Geometry check sheet. Reference: the model listing, model coordinates, mm. A direction names the side the tool comes from. Coordinates: 2 decimals unless noted, no trailing zeros. Write each loop counter-clockwise with the first axis right and the second up, starting at its lowest first coordinate (ties: lowest second). Pieces come first, ordered by that corner, then holes. Notation, with made-up numbers: (-27, 15.25) -> (-23, 15.25) arc R16 ccw to (-23, 34.25) -> close; hole circle Ø9 at (84.25, 15.5). An arc over 180 degrees is marked (long way). One line per question, with ' | ' between items.
Autodesk Inventor part; units mm, degrees
ref_plane "YZ Plane" through (0, 0, 0) normal (1, 0, 0) x (0, 1, 0)
ref_plane "XZ Plane" through (0, 0, 0) normal (0, 1, 0) x (-1, 0, 0)
ref_plane "XY Plane" through (0, 0, 0) normal (0, 0, 1) x (1, 0, 0)
sketch "Sketch1" plane through (0, 0, 0) normal (0, 0, 1) x (1, 0, 0)
  line L0 (-16.5, -70) -> (16.5, -70)
  line L1 (16.5, -70) -> (16.5, 70)
  line L2 (16.5, 70) -> (-16.5, 70)
  line L3 (-16.5, 70) -> (-16.5, -70)
  line L4 (-16.5, -70) -> (16.5, 70) construction
  line L5 (16.5, -70) -> (-16.5, 70) construction
  line L6 (0, 70) -> (0, -70)
  line L7 (11.5, 30) -> (14.5, 30)
  line L8 (14.5, 30) -> (14.5, -30)
  line L9 (14.5, -30) -> (11.5, -30)
  line L10 (11.5, -30) -> (11.5, 30)
  line L11 (-11.5, 30) -> (-14.5, 30)
  line L12 (-14.5, -30) -> (-11.5, -30)
  line L13 (-14.5, 30) -> (-14.5, -30)
  line L14 (-11.5, -30) -> (-11.5, 30)
  circle A0 centre (0, -60) radius 1.7
  circle A1 centre (0, 56) radius 10
  line L15 (-10, 56) -> (10, 56)
  line L16 (-6.3196, 63.75) -> (6.3196, 63.75)
  line L17 (-6.3196, 48.25) -> (6.3196, 48.25)
  circle A2 centre (8.75, 36) radius 1.65
  circle A3 centre (-8.75, 36) radius 1.65
  circle A4 centre (0, 56) radius 4
  point P0 (0, 0)
  point P1 (0, 0)
  point P2 (14.5, 0)
  point P3 (16.5, 0)
  point P4 (-14.5, 0)
  point P5 (0, 0)
  point P6 (-6.3196, 48.25)
  point P7 (6.3196, 48.25)
  dimension "d0" = 140
  dimension "d1" = 3
  dimension "d2" = 2
  dimension "d3" = 60
  dimension "d6" = 3.4
  dimension "d7" = 10
  dimension "d9" = 23
  dimension "d13" = 14
  dimension "d14" = 20
  dimension "d15" = 15.5
  dimension "d17" = 3.3
  dimension "d18" = 20
  dimension "d19" = 17.5
  dimension "d22" = 8
extrude "Plate1" add sketch "Sketch1" along normal blind 3 contours L3 L2 L6 A1 A0 L0 | L6 A0 A1 L2 L1 L0 | A1 L16 L6 | L6 L16 A1 | A1 L17 L6 | L6 L17 A1 | L16 A1 L15 A4 L6 | L6 A4 L15 A1 L16 | L17 A1 L15 A4 L6 | L6 A4 L15 A1 L17
sketch "Sketch3" plane through (0, 0, 3) normal (0, 0, 1) x (1, 0, 0)
  line L0 (-16.5, 70) -> (-16.5, -70)
  line L1 (-16.5, 70) -> (16.5, 70)
  line L2 (16.5, 70) -> (16.5, 90)
  line L3 (16.5, 90) -> (-16.5, 90)
  line L4 (-16.5, 90) -> (-16.5, 70)
  line L5 (-16.5, 0) -> (16.5, 0)
  line L6 (16.5, -70) -> (16.5, 70)
  point P0 (0, 0)
  dimension "d23" = 20
sheet face with bend "Face2" sketch "Sketch3" thickness 3 toward (0, 0, -1) bend radius 3 contours L4 L3 L2 L1
bend "Bend1"
sketch "Sketch4" plane through (0, 0, 3) normal (0, 0, 1) x (1, 0, 0)
  line L0 (-10, -70) -> (10, -70)
  line L1 (10, -70) -> (10, -75)
  line L2 (10, -75) -> (-10, -75)
  line L3 (-10, -75) -> (-10, -70)
  line L4 (16.5, -70) -> (-16.5, -70)
  point P0 (0, 0)
  point P1 (0, -70)
  point P2 (0, -70)
  point P3 (0, -70)
  dimension "d29" = 20
  dimension "d30" = 5
sheet face with bend "Face3" sketch "Sketch4" thickness 3 toward (0, 0, -1) bend radius 3
bend "Bend2"
sketch "Sketch5" plane through (0, 0, 3) normal (0, 0, 1) x (1, 0, 0)
  line L0 (-3, 23.5) -> (3, 23.5)
  line L1 (3, 23.5) -> (3, 28.5)
  line L2 (3, 28.5) -> (-3, 28.5)
  line L3 (-3, 28.5) -> (-3, 23.5)
  line L4 (-3, 23.5) -> (3, 28.5) construction
  line L5 (3, 23.5) -> (-3, 28.5) construction
  circle A0 centre (0, 56) radius 4
  point P0 (0, 0)
  point P1 (0, 26)
  dimension "d36" = 6
  dimension "d37" = 5
  dimension "d38" = 30
extrude "Cut1" cut sketch "Sketch5" against normal blind 3 contours L3 L2 L1 L0
sketch "Sketch6" plane through (0, 0, 3) normal (0, 0, 1) x (1, 0, 0)
  line L0 (-6.325, 78.95) -> (6.325, 78.95)
  line L1 (6.325, 78.95) -> (6.325, 73.05)
  line L2 (6.325, 73.05) -> (-6.325, 73.05)
  line L3 (-6.325, 73.05) -> (-6.325, 78.95)
  line L4 (-6.325, 78.95) -> (6.325, 73.05) construction
  line L5 (6.325, 78.95) -> (-6.325, 73.05) construction
  circle A0 centre (0, 56) radius 4
  point P0 (0, 0)
  point P1 (0, 76)
  dimension "d41" = 12.65
  dimension "d42" = 5.9
  dimension "d43" = 20
extrude "Cut2" cut sketch "Sketch6" against normal blind 3 contours L0 L1 L2 L3
equation "\"d39\" = Thickness"
equation "\"d44\" = Thickness"
equation "\"d16\" = Thickness"
equation "\"d24\" = BendRadius"
equation "\"d25\" = BendReliefWidth"
equation "\"d27\" = MinimumRemnant"
equation "\"d26\" = BendReliefDepth"
equation "\"d28\" = TransitionRadius"
equation "\"d31\" = BendRadius"
equation "\"d32\" = BendReliefWidth"
equation "\"d34\" = MinimumRemnant"
equation "\"d33\" = BendReliefDepth"
equation "\"d35\" = TransitionRadius"
equation "\"BendRadius\" = Thickness"
equation "\"BendReliefWidth\" = Thickness"
equation "\"BendReliefDepth\" = 0.5 * Thickness"
equation "\"CornerReliefSize\" = 4 * Thickness"
equation "\"MinimumRemnant\" = 2 * Thickness"
equation "\"TransitionRadius\" = BendRadius"
equation "\"JacobiRadiusSize\" = BendRadius"
equation "\"GapSize\" = Thickness"
properties part number "Motor Fixation .1 FV"
1. Material ranges on line 1 (Y direction, x = 0, z = 0.9); line 2 (X direction, y = 17.5, z = 1.1); line 3 (X direction, y = 56, z = 0.6), recorded low to high. Write a range as from..to.
Worked answers:
line 1: -75..-61.7, -58.3..23.5, 28.5..52, 60..73.05, 78.95..90 | line 2: -16.5..-14.5, -11.5..11.5, 14.5..16.5 | line 3: -16.5..-4, 4..16.5
2. Cross-section at C-C on z = 1.5. Give the number of separate pieces and of enclosed holes in the cut face, and give its area (3 significant figures).
Worked answers:
separate pieces: 1 | enclosed holes: 8 | area: 4,840 mm²
3. Cross-section at B-B on y = 56. Record the boundary of the cut face in (x, z), and give its area (3 significant figures).
Worked answers:
outline: (-16.5, 0) -> (-4, 0) -> (-4, 3) -> (-16.5, 3) -> close; (4, 0) -> (16.5, 0) -> (16.5, 3) -> (4, 3) -> close | area: 75.0 mm²
4. Cross-section at A-A on x = 0. Record the boundary of the cut face in (y, z).
Worked answers:
outline: (-75, 0) -> (-61.7, 0) -> (-61.7, 3) -> (-75, 3) -> close; (-58.3, 0) -> (23.5, 0) -> (23.5, 3) -> (-58.3, 3) -> close; (28.5, 0) -> (52, 0) -> (52, 3) -> (28.5, 3) -> close; (60, 0) -> (73.05, 0) -> (73.05, 3) -> (60, 3) -> close; (78.95, 0) -> (90, 0) -> (90, 3) -> (78.95, 3) -> close
5. Tool access check on faces 4 (the face through (-13, -30, 1)), 5 (the face through (-10, -73, 2)), 6 (the face through (0, 90, 2)). Record the directions out of +Z, -Z, +X, -X, +Y, -Y that give a thin tool (end or side, any length) a straight path to the whole face; none if there is none.
Worked answers:
face 4: +Z, -Z | face 5: +Z, -Z, -X, -Y | face 6: +Z, -Z, +X, -X, +Y
6. Mould release check, pull along Y, two halves, no side actions. Record for faces 1 (the face through (9.64, 34.61, 1.48)), 2 (the face through (0, 9, 0)), 3 (the face through (13, -70, 1)): released by +Y, released by -Y, zero draft, split by the parting line, or undercut.
Worked answers:
face 1: undercut | face 2: zero draft | face 3: released by -Y
7. Go/stop test with flat-tipped pins: P1, Ø5, axis at x = 0, y = 56, coming from the +Z side; P2, Ø0.9, axis at x = 12, z = 1, coming from the -Y side; P3, Ø10, axis at x = 1, y = -55.5, coming from the -Z side. Record where each tip stops, or that it passes through.
Worked answers:
P1: through | P2: y = -70 | P3: z = 0
8. Cross-section at D-D on y = 36. Record the boundary of the cut face in (x, z).
Worked answers:
outline: (-16.5, 0) -> (-10.4, 0) -> (-10.4, 3) -> (-16.5, 3) -> close; (-7.1, 0) -> (7.1, 0) -> (7.1, 3) -> (-7.1, 3) -> close; (10.4, 0) -> (16.5, 0) -> (16.5, 3) -> (10.4, 3) -> close
